Here's the drawing with two shaded views (mm, measured from the low corner). I have some questions. A direction names the side the tool comes from. Round coordinates to 2 decimals unless told otherwise and drop trailing zeros. Loops run counter-clockwise (first coordinate to the right, second up) from the corner with the lowest first, then second, coordinate; pieces in that order, holes last.
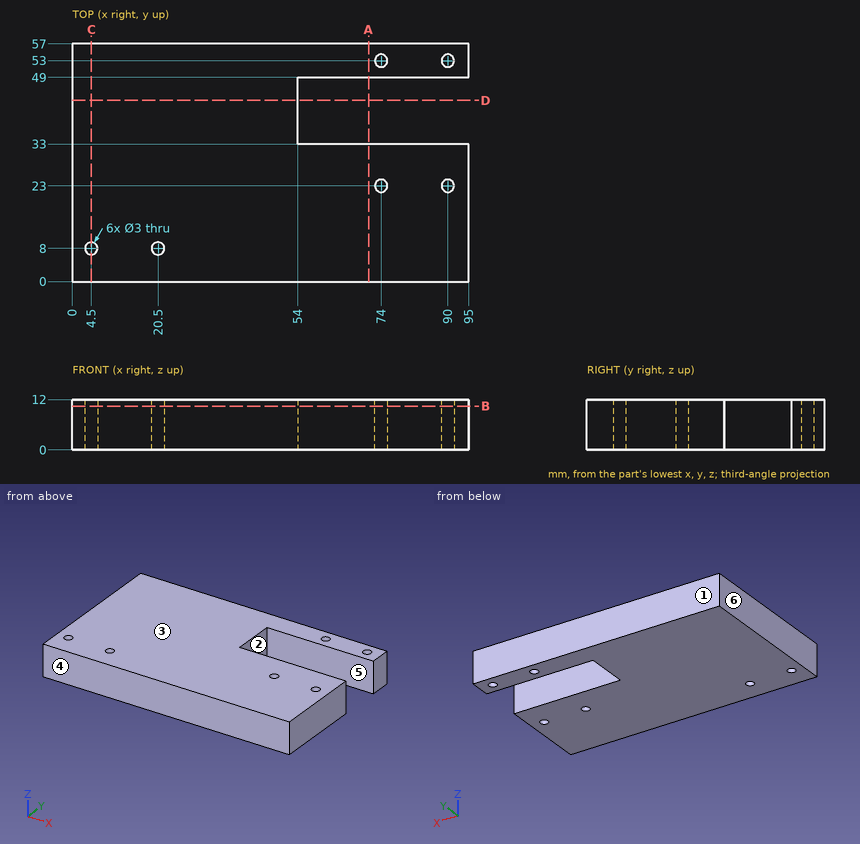
(1) If we section it at C-C, the plane x = 4.5: List the corners of the cut face in (y, z) for me, then the cut area to 3 significant figures.
Worked answers:
outline: (0, 0) - (6.5, 0) - (6.5, 12) - (0, 12) - close; (9.5, 0) - (57, 0) - (57, 12) - (9.5, 12) - close
area: 648 mm2
(2) If we section it at D-D, the plane y = 43.5: List the corners of the cut face in (x, z) for me.
Worked answers:
outline: (0, 0) - (54, 0) - (54, 12) - (0, 12) - close
(3) For the marked faces 5 and 6, which set-ups out of +Z, -Z, +X, -X, +Y, -Y let a thin tool reach every point of the face, with its end or its side?
Worked answers:
face 5: +Z, -Z, +X
face 6: +Z, -Z, -X, +Y, -Y
(4) If we section it at A-A, the plane x = 71: List the corners of the cut face in (y, z) for me, then the cut area to 3 significant figures.
Worked answers:
outline: (0, 0) - (33, 0) - (33, 12) - (0, 12) - close; (49, 0) - (57, 0) - (57, 12) - (49, 12) - close
area: 492 mm2
(5) If we section it at B-B, the plane z = 10.5: List the corners of the cut face in (x, y) for me.
Worked answers:
outline: (0, 0) - (95, 0) - (95, 33) - (54, 33) - (54, 49) - (95, 49) - (95, 57) - (0, 57) - close; hole circle Ø3 at (4.5, 8); hole circle Ø3 at (20.5, 8); hole circle Ø3 at (74, 23); hole circle Ø3 at (74, 53); hole circle Ø3 at (90, 23); hole circle Ø3 at (90, 53)
(6) If we mould it in two halves opening along Y, with no side actions, what happens to the marked faces 1, 2, 3 and 4? For each: released by +Y, released by -Y, zero draft, split by the parting line, or undercut.
Worked answers:
face 1: released by +Y
face 2: undercut
face 3: zero draft
face 4: released by -Y
(7) If I drill on line 1 (Y direction, x = 90, z = 8.5); line 2 (Y direction, x = 67, z = 0.5); line 3 (X direction, y = 7.5, z = 2.75), over which ranges is the centre line in solid material (lowest first)?
Worked answers:
line 1: y = 0 to 21.5, 24.5 to 33, 49 to 51.5, 54.5 to 57
line 2: y = 0 to 33, 49 to 57
line 3: x = 0 to 3.09, 5.91 to 19.09, 21.91 to 95
